Part print with two shaded views. Sizes in mm from the minimum x, y, z corner. Round coordinates to 2 decimals unless told otherwise and drop trailing zeros. Write each loop counter-clockwise with the first axis right and the second up, starting at its lowest first coordinate (ties: lowest second). Pieces come first, ordered by that corner, then holes.
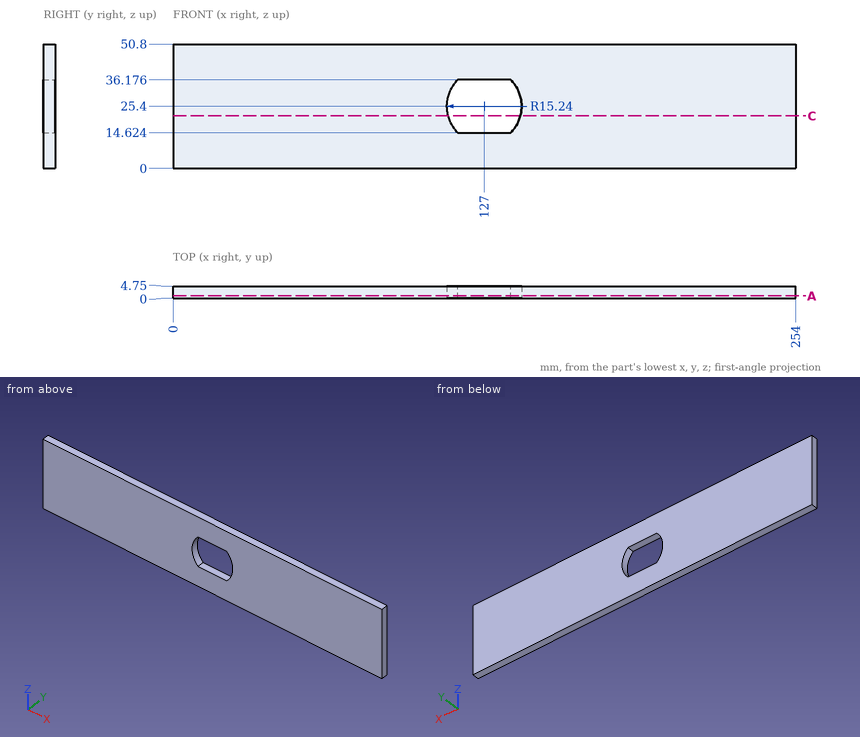
Q1. Cut at C-C on z = 21.5. Write the cut outline in (x, y), plus the area to 3 significant figures.
Values follow:
outline: (0, 0) - (112.27, 0) - (112.27, 4.75) - (0, 4.75) - close; (141.73, 0) - (254, 0) - (254, 4.75) - (141.73, 4.75) - close
area: 1,070 mm2
Q2. Wall check: L1, parallel to X at y = 1.25, z = 26; L2, parallel to Z at x = 127, y = 1.25; L3, parallel to X at y = 2.5, z = 29. Give the ranges that are in metal, low to high.
Values follow:
L1: x = 0 to 111.77, 142.23 to 254
L2: z = 0 to 14.62, 36.18 to 50.8
L3: x = 0 to 112.19, 141.81 to 254
Q3. Cut at A-A on y = 0.9. Write the cut outline in (x, z).
Values follow:
outline: (0, 0) - (254, 0) - (254, 50.8) - (0, 50.8) - close; hole (116.22, 14.62) - (137.78, 14.62) arc R15.24 ccw to (137.78, 36.18) - (116.22, 36.18) arc R15.24 ccw to start
